For this review, take the finished solid that the model builds, in its own axes (mm). A direction names the side the tool comes from. Give positions to 0.01 mm unless a question says otherwise; leave off trailing zeros. Write each loop counter-clockwise with the first axis right and the second up, starting at its lowest first coordinate (ties: lowest second). Pieces come first, ordered by that corner, then holes.
from build123d import *

# Parameters (mm, degrees)
SKETCH1_R               = 10.95
SKETCH1_R_2             = 6.05
BOSS_EXTRUDE1_DEPTH     = 2
BOSS_EXTRUDE2_START     = 12
SKETCH1_3_R             = 10.95
SKETCH1_3_R_2           = 6.05
BOSS_EXTRUDE2_DEPTH     = 12
BOSS_EXTRUDE3_START     = -2.5
SKETCH2_R               = 12.95
SKETCH2_R_2             = 10.95
BOSS_EXTRUDE3_DEPTH     = 11.5
CUT_EXTRUDE1_DEPTH      = 22.895319134
CUT_EXTRUDE1_DEPTH_BACK = 22.895319134
SKETCH3_W               = 100
SKETCH3_H               = 23
CUT_EXTRUDE3_DEPTH      = 22.07018035
CUT_EXTRUDE3_DEPTH_BACK = 22.07018035
BOSS_EXTRUDE4_START     = 12
SKETCH1_5_R             = 10.95
SKETCH1_5_R_2           = 6.05
BOSS_EXTRUDE4_DEPTH     = 12
SKETCH5_W               = 18
SKETCH5_H               = 4
CUT_EXTRUDE4_DEPTH      = 22.07018035
FILLET1_R               = 2
CUT_EXTRUDE5_DEPTH      = 22.070180523
CUT_EXTRUDE5_DEPTH_BACK = 22.070180523
SKETCH6_R               = 1.6
CHAMFER1_SIZE           = 1


# Some blends are built 0.0001 mm under size
with BuildPart() as part:
    # Sketch1 → Boss-Extrude1 (new body)
    # profile 1 of 2: a face of its own
    with BuildSketch(Plane(origin=(0, 0, 0), x_dir=(1, 0, 0), z_dir=(0, 1, 0))):
        with Locations(Location((0, 0, 0), (0, 0, 270))):
            Circle(SKETCH1_R)
        Circle(SKETCH1_R_2, mode=Mode.SUBTRACT)
    # profile 2 of 2: a face of its own
    with BuildSketch(Plane(origin=(0, 0, 0), x_dir=(1, 0, 0), z_dir=(0, 1, 0))):
        Circle(SKETCH1_R_2)
    extrude(amount=-BOSS_EXTRUDE1_DEPTH)

    # Sketch1<3> → Boss-Extrude2 (add)
    with BuildSketch(Plane(origin=(0, 0, 0), x_dir=(1, 0, 0), z_dir=(0, 1, 0)).offset(BOSS_EXTRUDE2_START)):
        with Locations(Location((0, 0, 0), (0, 0, 270))):
            Circle(SKETCH1_3_R)
        with Locations(Location((0, 0, 0), (0, 0, 270))):
            Circle(SKETCH1_3_R_2, mode=Mode.SUBTRACT)
    extrude(amount=-BOSS_EXTRUDE2_DEPTH)

    # Sketch2 → Boss-Extrude3 (add)
    with BuildSketch(Plane(origin=(0, 12, 0), x_dir=(1, 0, 0), z_dir=(0, 1, 0)).offset(BOSS_EXTRUDE3_START)):
        with Locations(Location((0, 0, 0), (0, 0, 270))):
            Circle(SKETCH2_R)
        with Locations(Location((0, 0, 0), (0, 0, 270))):
            Circle(SKETCH2_R_2, mode=Mode.SUBTRACT)
    extrude(amount=-BOSS_EXTRUDE3_DEPTH)

    # Sketch3 → Cut-Extrude1 (cut, two sides: drawn at the far end of the back side and taken through both)
    with BuildSketch(Plane(origin=(0, 0, 0), x_dir=(1, 0, 0), z_dir=(0, 1, 0)).offset(-CUT_EXTRUDE1_DEPTH_BACK)):
        with Locations((0, -23)):
            Rectangle(SKETCH3_W, SKETCH3_H)
        with Locations((0, 23)):
            Rectangle(SKETCH3_W, SKETCH3_H)
    extrude(amount=CUT_EXTRUDE1_DEPTH + CUT_EXTRUDE1_DEPTH_BACK, mode=Mode.SUBTRACT)

    # Sketch4 → Cut-Extrude3 (cut, two sides: drawn at the far end of the back side and taken through both)
    with BuildSketch(Plane.XY.offset(-CUT_EXTRUDE3_DEPTH_BACK)):
        Polygon((13, 12), (4.5, 12), (13, 3.5), align=None)
    extrude(amount=CUT_EXTRUDE3_DEPTH + CUT_EXTRUDE3_DEPTH_BACK, mode=Mode.SUBTRACT)

    # Sketch1<5> → Boss-Extrude4 (add)
    with BuildSketch(Plane(origin=(0, 0, 0), x_dir=(1, 0, 0), z_dir=(0, 1, 0)).offset(BOSS_EXTRUDE4_START)):
        with Locations(Location((0, 0, 0), (0, 0, 270))):
            Circle(SKETCH1_5_R)
        with Locations(Location((0, 0, 0), (0, 0, 270))):
            Circle(SKETCH1_5_R_2, mode=Mode.SUBTRACT)
    extrude(amount=-BOSS_EXTRUDE4_DEPTH)

    # Sketch5 → Cut-Extrude4 (cut, through all)
    with BuildSketch(Plane(origin=(0, 0, 0), x_dir=(1, 0, 0), z_dir=(0, 1, 0))):
        with Locations((-11, 0)):
            Rectangle(SKETCH5_W, SKETCH5_H)
    extrude(amount=CUT_EXTRUDE4_DEPTH, mode=Mode.SUBTRACT)

    # Fillet1
    fillet1_edges = [part.edges().sort_by_distance(p)[0] for p in [
        (-8.237831116, 12, 2),
        (-8.237831116, 12, -2),
        (-9.252243836, 0, -2),
        (-9.252243836, 0, 2),
    ]]
    fillet(fillet1_edges, radius=FILLET1_R - 0.0001)  # a hair under: the kernel refuses the full size

    # Sketch6 → Cut-Extrude5 (cut, two sides: drawn at the far end of the back side and taken through both)
    with BuildSketch(Plane(origin=(0, 0, 0), x_dir=(1, 0, 0), z_dir=(0, 1, 0)).offset(-CUT_EXTRUDE5_DEPTH_BACK)):
        with Locations(Location((0, 0, 0), (0, 0, 270))):
            Circle(SKETCH6_R)
    extrude(amount=CUT_EXTRUDE5_DEPTH + CUT_EXTRUDE5_DEPTH_BACK, mode=Mode.SUBTRACT)

    # Chamfer1
    # the kernel refuses this chamfer: 1 mm, written as the material it takes off along each edge
    with BuildSketch(Plane(origin=(8.525883186, 9.5, 11.5), x_dir=(0, 0.027495876610585647, -0.9996219169112968), z_dir=(-1, 0, 0))) as chamfer1_piece_1_section:
        Polygon((CHAMFER1_SIZE * 0.999621916911, CHAMFER1_SIZE * 0.0274958766106), (-CHAMFER1_SIZE * 0.0274958766106, CHAMFER1_SIZE * 0.999621916911), (0, 0), align=None)
    chamfer1_piece_1 = extrude(amount=17.051766372, mode=Mode.PRIVATE)
    chamfer1_piece_1 = chamfer1_piece_1 - Plane(origin=(0, 9.159933663, 0), x_dir=(0, 0, 1), z_dir=(0, 1, 0)) * Cylinder(10.95, 39, mode=Mode.PRIVATE)
    add(chamfer1_piece_1, mode=Mode.SUBTRACT)
    with BuildSketch(Plane(origin=(8.525883186, 9.5, -11.5), x_dir=(0, 0.027495876610585647, 0.9996219169112968), z_dir=(-1, 0, 0))) as chamfer1_piece_2_section:
        Polygon((CHAMFER1_SIZE * 0.999621916911, -CHAMFER1_SIZE * 0.0274958766106), (-CHAMFER1_SIZE * 0.0274958766106, -CHAMFER1_SIZE * 0.999621916911), (0, 0), align=None)
    chamfer1_piece_2 = extrude(amount=17.051766372, mode=Mode.PRIVATE)
    chamfer1_piece_2 = chamfer1_piece_2 - Plane(origin=(0, 9.159933662, 0), x_dir=(0, 0, 1), z_dir=(0, 1, 0)) * Cylinder(10.95, 39, mode=Mode.PRIVATE)
    add(chamfer1_piece_2, mode=Mode.SUBTRACT)


solid = part.part
(1) We need section A-A (x = 0). Write out the cut boundary in (y, z).
(2) We need section C-C (y = 7.75). Write out the cut boundary in (x, z), and give its area (3 significant figures).
(3) Tool access review of faces 4 (the flat face through (11.3, 5.2, -0.2)), 5 (the flat face through (-9, 6, -2)), 6 (the flat face through (6, 9.5, -10)): name each direction out of +Z, -Z, +X, -X, +Y, -Y from which nothing blocks a thin tool from reaching the whole face with its end or side.
(4) Clearance check with flat-ended pins moving along their axes: pin 1 Ø5.5 at (x, y) = (-10, 8) entering from +Z; pin 2 Ø4 at (x, z) = (0, 0) entering from +Y; pin 3 Ø1.5 at (y, z) = (2, -2.5) entering from +X. State where each tip first meets the part, or that it passes through.
(5) We need section B-B (z = -1.25). Write out the cut boundary in (x, y), and give its area (3 significant figures).
(6) For L1, parallel to X at y = -0.55, z = 0; L2, parallel to Z at x = 0, y = -0.95; L3, parallel to X at y = 10.75, z = 5.25, list the stretches that pass through material, from the lowest coordinate up.
(7) The part is to be moulded in two halves that separate along Z. For faces 1 (the cylindrical face through (-9.28, 0.57, 1.4)), 2 (the flat face through (0, 3, -11.5)), 3 (the flat face through (-0.1, 8.9, 11.1)), say which applies: +Z half, -Z half, draft (parallel to the pull), parting line (faces both ways), or undercut.
The answers:
1. outline: (-2, -11.5) - (8.5, -11.5) - (9.05, -10.95) - (12, -10.95) - (12, -6.05) - (0, -6.05) - (0, -1.6) - (-2, -1.6) - close; (-2, 1.6) - (0, 1.6) - (0, 6.05) - (12, 6.05) - (12, 10.95) - (9.05, 10.95) - (8.5, 11.5) - (-2, 11.5) - close
2. outline: (-12.79, -2) arc R12.95 ccw to (-5.95, -11.5) - (5.95, -11.5) arc R12.95 ccw to (8.75, -9.55) - (8.75, -6.58) arc R10.95 ccw to (8.75, 6.58) - (8.75, 9.55) arc R12.95 ccw to (5.95, 11.5) - (-5.95, 11.5) arc R12.95 ccw to (-12.79, 2) - (-5.71, 2) arc R6.05 cw (long way) to (-5.71, -2) - close
2. area: 325 mm2
3. face 4: +X, +Y
3. face 5: -X, +Y
3. face 6: -Z, +X, +Y
4. pin 1: stops at z = 10.73
4. pin 2: stops at y = 0
4. pin 3: stops at x = 12.83
5. outline: (-12.89, -2) - (-1, -2) - (-1, 0) - (-5.92, 0) - (-5.92, 0.44) - (-12.89, 0.44) - close; (1, -2) - (12.89, -2) - (12.89, 3.61) - (10.88, 5.62) - (10.88, 12) - (5.92, 12) - (5.92, 0) - (1, 0) - close
5. area: 119 mm2
6. L1: x = -12.95 to -1.6, 1.6 to 12.95
6. L2: z = -11.5 to -1.6, 1.6 to 11.5
6. L3: x = -9.61 to -3.01, 3.01 to 9.61
7. face 1: undercut
7. face 2: -Z half
7. face 3: +Z half
